Check sheet for the modelled part. Datum: model origin and axes. Units: mm. Face numbers are marked on the shaded views. A direction names the side the tool comes from. Give positions to 0.01 mm unless a question says otherwise; leave off trailing zeros. Write each loop counter-clockwise with the first axis right and the second up, starting at its lowest first coordinate (ties: lowest second). Pieces come first, ordered by that corner, then holes. Notation, with made-up numbers: (81.25, 43) -> (113.25, 43) arc R11 cw to (113.25, 62) -> close; hole circle Ø11 at (27.5, 70.25). An arc over 180 degrees is marked (long way). Return JSON: item names as keys, results as strings.
from build123d import *

# Parameters (mm, degrees)
SKETCH2_W           = 93.98
SKETCH2_H           = 66.04
BOSS_EXTRUDE1_DEPTH = 17.78
SKETCH3_W           = 93.98
SKETCH3_H           = 5.588
BOSS_EXTRUDE2_DEPTH = 12.7
SKETCH4_W           = 82.55
SKETCH4_H           = 9.525
SKETCH4_W_2         = 76.2
SKETCH4_H_2         = 3.175
CUT_EXTRUDE1_DEPTH  = 60.452
SKETCH5_W           = 93.98
SKETCH5_H           = 5.588
BOSS_EXTRUDE3_DEPTH = 12.7
SKETCH6_R           = 2.413
SKETCH6_R_2         = 3.81
CUT_EXTRUDE2_DEPTH  = 116.826228049
FILLET1_R           = 1.27
FILLET2_R           = 1.27
FILLET3_R           = 1.27


with BuildPart() as part:
    # Sketch2 → Boss-Extrude1 (new body)
    with BuildSketch(Plane.XY):
        with Locations((46.99, 33.02)):
            Rectangle(SKETCH2_W, SKETCH2_H)
    extrude(amount=BOSS_EXTRUDE1_DEPTH)

    # Sketch3 → Boss-Extrude2 (add)
    with BuildSketch(Plane.XY.offset(17.78)):
        with Locations((46.99, 2.794)):
            Rectangle(SKETCH3_W, SKETCH3_H)
    extrude(amount=BOSS_EXTRUDE2_DEPTH)

    # Sketch4 → Cut-Extrude1 (cut)
    with BuildSketch(Plane(origin=(0, 66.04, 0), x_dir=(1, 0, 0), z_dir=(0, 1, 0))):
        with Locations((46.99, -9.8425)):
            Rectangle(SKETCH4_W, SKETCH4_H)
        with Locations((46.99, -16.1925)):
            Rectangle(SKETCH4_W_2, SKETCH4_H_2)
    extrude(amount=-CUT_EXTRUDE1_DEPTH, mode=Mode.SUBTRACT)

    # Sketch5 → Boss-Extrude3 (add)
    with BuildSketch(Plane(origin=(0, 0, 0), x_dir=(-1, 0, 0), z_dir=(0, 0, -1))):
        with Locations((-46.99, 2.794)):
            Rectangle(SKETCH5_W, SKETCH5_H)
    extrude(amount=BOSS_EXTRUDE3_DEPTH)

    # Sketch6 → Cut-Extrude2 (cut, through all)
    with BuildSketch(Plane(origin=(0, 5.588, 0), x_dir=(1, 0, 0), z_dir=(0, 1, 0))):
        with Locations(Location((8.89, 6.35, 0), (0, 0, 270))):
            Circle(SKETCH6_R)
        with Locations(Location((21.59, 6.35, 0), (0, 0, 270))):
            Circle(SKETCH6_R)
        with Locations(Location((34.29, 6.35, 0), (0, 0, 270))):
            Circle(SKETCH6_R)
        with Locations(Location((46.99, 6.35, 0), (0, 0, 270))):
            Circle(SKETCH6_R)
        with Locations(Location((59.69, 6.35, 0), (0, 0, 270))):
            Circle(SKETCH6_R)
        with Locations(Location((72.39, 6.35, 0), (0, 0, 270))):
            Circle(SKETCH6_R)
        with Locations(Location((85.09, 6.35, 0), (0, 0, 270))):
            Circle(SKETCH6_R)
        with Locations(Location((8.89, -22.86, 0), (0, 0, 270))):
            Circle(SKETCH6_R_2)
        with Locations(Location((24.13, -22.86, 0), (0, 0, 270))):
            Circle(SKETCH6_R_2)
        with Locations(Location((39.37, -22.86, 0), (0, 0, 270))):
            Circle(SKETCH6_R_2)
        with Locations(Location((54.61, -22.86, 0), (0, 0, 270))):
            Circle(SKETCH6_R_2)
        with Locations(Location((69.85, -22.86, 0), (0, 0, 270))):
            Circle(SKETCH6_R_2)
        with Locations(Location((85.09, -22.86, 0), (0, 0, 270))):
            Circle(SKETCH6_R_2)
    extrude(amount=-CUT_EXTRUDE2_DEPTH, mode=Mode.SUBTRACT)

    # Fillet1
    fillet1_edges = [part.edges().sort_by_distance(p)[0] for p in [
        (89.535, 66.04, 17.78),
        (4.445, 66.04, 17.78),
        (88.265, 66.04, 9.8425),
        (46.99, 66.04, 5.08),
        (5.715, 66.04, 9.8425),
        (7.3025, 66.04, 14.605),
        (8.89, 66.04, 16.1925),
        (86.6775, 66.04, 14.605),
        (85.09, 66.04, 16.1925),
        (46.99, 66.04, 0),
        (0, 66.04, 8.89),
        (93.98, 66.04, 8.89),
    ]]
    fillet(fillet1_edges, radius=FILLET1_R)

    # Fillet2
    fillet2_edges = [part.edges().sort_by_distance(p)[0] for p in [
        (0, 5.588, 24.13),
        (93.98, 5.588, 24.13),
        (46.99, 5.588, 30.48),
        (93.98, 5.588, -6.35),
        (0, 5.588, -6.35),
        (46.99, 5.588, -12.7),
    ]]
    fillet(fillet2_edges, radius=FILLET2_R)

    # Fillet3
    fillet3_edges = [part.edges().sort_by_distance(p)[0] for p in [
        (46.99, 0, 30.48),
        (46.99, 0, -12.7),
        (93.98, 0, 8.89),
        (0, 0, 8.89),
    ]]
    fillet(fillet3_edges, radius=FILLET3_R)


solid = part.part
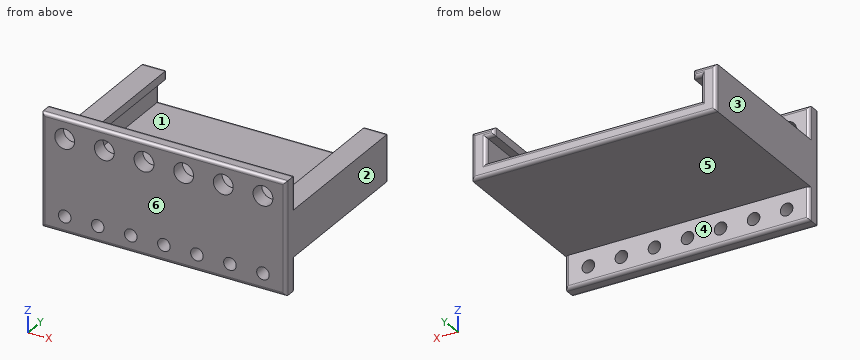
(1) Depth check by flat-ended pin: pin 1 Ø3 at (x, y) = (80.5, 27.5) entering from -Z; pin 2 Ø3.5 at (x, z) = (34, -3) entering from +Y; pin 3 Ø2.5 at (x, y) = (88, 31) entering from +Z; pin 4 Ø4 at (x, z) = (34.29, -6.35) entering from +Y. Enter the tip coordinate at first touch or a pass-through.
Reply:
{"pin 1": "z = 0", "pin 2": "y = 5.59", "pin 3": "z = 17.78", "pin 4": "through"}
(2) Cross-section at D-D on z = 10.5. Enter the section's corners in (x, y) (3 decimals).
Reply:
{"outline": "(0, 1.27) arc R1.27 ccw to (1.27, 0) -> (92.71, 0) arc R1.27 ccw to (93.98, 1.27) -> (93.98, 64.77) arc R1.27 ccw to (92.71, 66.04) -> (89.535, 66.04) arc R1.27 ccw to (88.265, 64.77) -> (88.265, 5.588) -> (5.715, 5.588) -> (5.715, 64.77) arc R1.27 ccw to (4.445, 66.04) -> (1.27, 66.04) arc R1.27 ccw to (0, 64.77) -> close"}
(3) Thickness scan on L1, parallel to X at y = 62.5, z = 9.5 (3 decimals); L2, parallel to Z at x = 88, y = 58 (3 decimals); L3, parallel to Y at x = 49, z = 28.5. Record the ranges inside material, lowest first.
Reply:
{"L1": "0 to 5.715, 88.265 to 93.98", "L2": "0 to 5.08, 14.605 to 17.78", "L3": "0 to 5.59"}
(4) Cross-section at B-B on y = 19. Enter the section's corners in (x, z) (3 decimals), then the cut area to 3 significant figures.
Reply:
{"outline": "(0, 0) -> (93.98, 0) -> (93.98, 17.78) -> (85.09, 17.78) -> (85.09, 14.605) -> (88.265, 14.605) -> (88.265, 5.08) -> (5.715, 5.08) -> (5.715, 14.605) -> (8.89, 14.605) -> (8.89, 17.78) -> (0, 17.78) -> close", "area": "643 mm^2"}
(5) Cross-section at C-C on x = 21.59. Enter the section's corners in (y, z).
Reply:
{"outline": "(0, -11.43) arc R1.27 ccw to (1.27, -12.7) -> (4.32, -12.7) arc R1.27 ccw to (5.59, -11.43) -> (5.59, -8.76) -> (0, -8.76) -> close; (0, -3.94) -> (5.59, -3.94) -> (5.59, 0) -> (64.77, 0) arc R1.27 ccw to (66.04, 1.27) -> (66.04, 3.81) arc R1.27 ccw to (64.77, 5.08) -> (5.59, 5.08) -> (5.59, 20.02) -> (0, 20.02) -> close; (0, 25.7) -> (5.59, 25.7) -> (5.59, 29.21) arc R1.27 ccw to (4.32, 30.48) -> (1.27, 30.48) arc R1.27 ccw to (0, 29.21) -> close"}
(6) Cross-section at A-A on x = 59.69. Enter the section's corners in (y, z), then the cut area to 3 significant figures.
Reply:
{"outline": "(0, -11.43) arc R1.27 ccw to (1.27, -12.7) -> (4.32, -12.7) arc R1.27 ccw to (5.59, -11.43) -> (5.59, -8.76) -> (0, -8.76) -> close; (0, -3.94) -> (5.59, -3.94) -> (5.59, 0) -> (64.77, 0) arc R1.27 ccw to (66.04, 1.27) -> (66.04, 3.81) arc R1.27 ccw to (64.77, 5.08) -> (5.59, 5.08) -> (5.59, 29.21) arc R1.27 ccw to (4.32, 30.48) -> (1.27, 30.48) arc R1.27 ccw to (0, 29.21) -> close", "area": "519 mm^2"}
(7) Set-up check for the marked faces 5 and 6: record each of +Z, -Z, +X, -X, +Y, -Y from which the full face is reachable in a straight line by a thin tool's end or side.
Reply:
{"face 5": "-Z, +X, -X, +Y", "face 6": "+Z, -Z, +X, -X, -Y"}
(8) Release check for a two-part mould opening along X. For the marked faces 1, 2, 3 and 4 record: pulls with the +X half, pulls with the -X half, needs draft (parallel to the pull), parting line crosses it, or undercut.
Reply:
{"face 1": "undercut", "face 2": "pulls with the +X half", "face 3": "pulls with the -X half", "face 4": "needs draft"}
